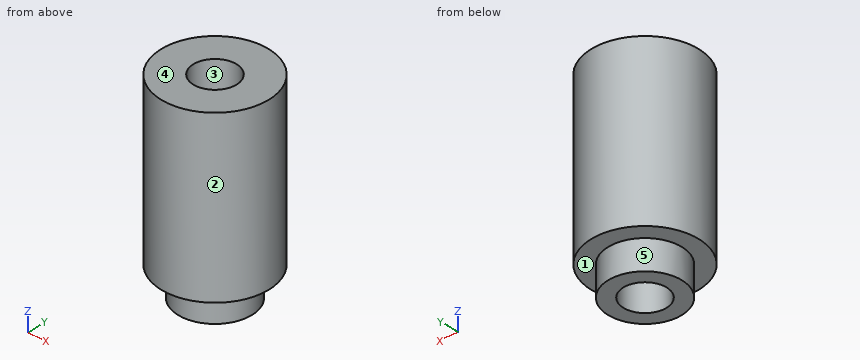
from build123d import *

# Parameters (mm, degrees)
MAIN_FEATURES_R          = 2.55
BODY_DEPTH               = 8
SKETCH1_3_R              = 1.75
PEG_DEPTH                = 1.4
M2_5X0_45_TAPPED_HOLE1_D = 2.05


with BuildPart() as part:
    # main_features → body (new body)
    with BuildSketch(Plane.XY):
        Circle(MAIN_FEATURES_R)
    extrude(amount=BODY_DEPTH)

    # Sketch1<3> → peg (add)
    with BuildSketch(Plane.XY):
        Circle(SKETCH1_3_R)
    extrude(amount=-PEG_DEPTH)

    # M2.5x0.45 Tapped Hole1 (through all)
    with Locations(Plane.XY.offset(8)):
        with Locations((0, 0)):
            Hole(M2_5X0_45_TAPPED_HOLE1_D / 2)


solid = part.part
Build history of the part. All positions in model axes, mm. Face numbers are marked on the shaded views. A direction names the side the tool comes from. Round coordinates to 2 decimals unless told otherwise and drop trailing zeros. Loops run counter-clockwise (first coordinate to the right, second up) from the corner with the lowest first, then second, coordinate; pieces in that order, holes last. Notation, with made-up numbers: (75, 85) -> (93, 85) arc R27 ccw to (93, 117) -> close; hole circle Ø10 at (-9.5, 81). An arc over 180 degrees is marked (long way). Use CSV: the item, a comma, the result in double quotes. Start each with the question number.
Q1. Saw through at A-A on x = 0. Give the cut face in (y, z) (3 decimals), and give its area (3 significant figures).
Q2. Drill centre lines: L1, parallel to Y at x = 0, z = 4.5 (3 decimals); L2, parallel to Z at x = 0.45, y = -2.05; L3, parallel to X at y = -0.7, z = 6.75. Where is each one in solid material? Low to high.
Q3. Mould opens along Y. For the marked faces 1, 2 and 3 say: +Y half, -Y half, draft (parallel to the pull), parting line (faces both ways), or undercut.
Q4. Saw through at C-C on z = 0.75. Give the cut face in (x, y) (3 decimals), and give its area (3 significant figures).
Q5. Saw through at D-D on y = -1.5. Give the cut face in (x, z), and give its area (3 significant figures).
Q6. Which spindle directions (+Z, -Z, +X, -X, +Y, -Y) get a long thin tool onto all of the face, cutting with end or side? Do the marked faces 4 and 5. Say none if no direction does.
Solutions:
1,outline,"(-2.55, 0) -> (-1.75, 0) -> (-1.75, -1.4) -> (-1.025, -1.4) -> (-1.025, 8) -> (-2.55, 8) -> close; (1.025, -1.4) -> (1.75, -1.4) -> (1.75, 0) -> (2.55, 0) -> (2.55, 8) -> (1.025, 8) -> close"
1,area,"26.4 mm^2"
2,L1,"y = -2.55 to -1.025, 1.025 to 2.55"
2,L2,"z = 0 to 8"
2,L3,"x = -2.45 to -0.75, 0.75 to 2.45"
3,face 1,"draft"
3,face 2,"parting line"
3,face 3,"undercut"
4,outline,"circle Ø5.1 at (0, 0); hole circle Ø2.05 at (0, 0)"
4,area,"17.1 mm^2"
5,outline,"(-2.06, 0) -> (-0.9, 0) -> (-0.9, -1.4) -> (0.9, -1.4) -> (0.9, 0) -> (2.06, 0) -> (2.06, 8) -> (-2.06, 8) -> close"
5,area,"35.5 mm^2"
6,face 4,"+Z, +X, -X, +Y, -Y"
6,face 5,"-Z"
